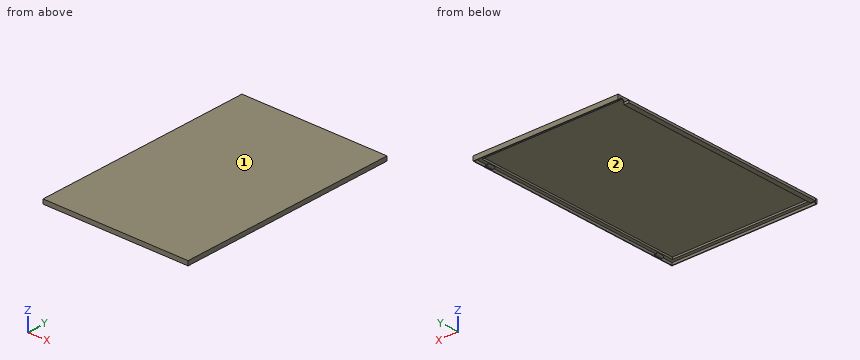
Autodesk Inventor part; units mm, degrees
ref_plane "DPB21_XY" through (247.5, 377.5, 0) normal (0, 0, 1) x (1, 0, 0)
ref_plane "DPB21_YZ" through (247.5, 377.5, 0) normal (1, 0, 0) x (0, 1, 0)
ref_plane "DPB21_ZX" through (247.5, 377.5, 0) normal (0, 1, 0) x (0, 0, 1)
sketch "Skizze_1" plane through (0, 0, 0) normal (0, 0, 1) x (1, 0, 0)
  line L0 (-247.5, 377.5) -> (-247.5, -377.5)
  line L1 (-247.5, -377.5) -> (247.5, -377.5)
  line L2 (247.5, -377.5) -> (247.5, 377.5)
  line L3 (247.5, 377.5) -> (-247.5, 377.5)
extrude "Extrusion1" add sketch "Skizze_1" against normal blind 15
sketch "Skizze_2" plane through (0, 0, 0) normal (1, 0, 0) x (0, 0, -1)
  line L0 (2, 375.5) -> (2, -375.5)
  line L1 (2, -375.5) -> (17, -375.5)
  line L2 (17, -375.5) -> (17, 375.5)
  line L3 (17, 375.5) -> (2, 375.5)
extrude "Extrusion2" cut sketch "Skizze_2" along normal mid plane 491
sketch "Skizze_3" plane through (0, 0, -2) normal (0, 0, 1) x (1, 0, 0)
  line L0 (-245.5, 361.5) -> (231.5, 361.5)
  line L1 (231.5, 361.5) -> (231.5, -361.5)
  line L2 (231.5, -361.5) -> (-245.5, -361.5)
  line L3 (-245.5, -361.5) -> (-245.5, -373.5)
  line L4 (-245.5, -373.5) -> (243.5, -373.5)
  line L5 (243.5, -373.5) -> (243.5, 373.5)
  line L6 (243.5, 373.5) -> (-245.5, 373.5)
  line L7 (-245.5, 373.5) -> (-245.5, 361.5)
sketch "Skizze_21" plane through (0, -320.6, 0) normal (0, 1, 0) x (1, 0, 0)
  arc A0 (240, 12.35) -> (240, 4.05) centre (240, 8.2) ccw
  line L0 (240, 4.05) -> (245.5, 4.05)
  line L1 (245.5, 4.05) -> (245.5, 5.5)
  line L2 (245.5, 5.5) -> (240, 5.5)
  arc A1 (240, 10.9) -> (240, 5.5) centre (240, 8.2) ccw
  line L3 (240, 10.9) -> (245.5, 10.9)
  line L4 (245.5, 10.9) -> (245.5, 12.35)
  line L5 (245.5, 12.35) -> (240, 12.35)
extrude "Extrusion3" add sketch "Skizze_21" along normal mid plane 26
sketch "Skizze_22" plane through (0, 320.6, 0) normal (0, 1, 0) x (1, 0, 0)
  arc A0 (240, 12.35) -> (240, 4.05) centre (240, 8.2) ccw
  line L0 (240, 4.05) -> (245.5, 4.05)
  line L1 (245.5, 4.05) -> (245.5, 5.5)
  line L2 (245.5, 5.5) -> (240, 5.5)
  arc A1 (240, 10.9) -> (240, 5.5) centre (240, 8.2) ccw
  line L3 (240, 10.9) -> (245.5, 10.9)
  line L4 (245.5, 10.9) -> (245.5, 12.35)
  line L5 (245.5, 12.35) -> (240, 12.35)
extrude "Extrusion4" add sketch "Skizze_22" along normal mid plane 26
sketch "Skizze_23" plane through (0, 0, 0) normal (0, 1, 0) x (1, 0, 0)
  line L0 (-263.5, 19) -> (-248, 19)
  arc A0 (-247.5, 18.5) -> (-248, 19) centre (-248, 18.5) ccw
  line L1 (-247.5, 18.5) -> (-247.5, 15)
  line L2 (-247.5, 15) -> (-245.5, 15)
  line L3 (-245.5, 15) -> (-245.5, 19.5)
  arc A1 (-245.5, 19.5) -> (-247, 21) centre (-247, 19.5) ccw
  line L4 (-247, 21) -> (-263.5, 21)
  line L5 (-263.5, 21) -> (-263.5, 19)
extrude "Extrusion5" add sketch "Skizze_23" along normal mid plane 707
sketch "Skizze_24" plane through (-247.5, 0, 0) normal (1, 0, 0) x (0, 0, -1)
  arc A0 (13.25, 372.2142) -> (15.5, 354.5) centre (15.5, 363.5) ccw
  line L0 (15.5, 354.5) -> (15.5, 375.119)
  arc A1 (13.25, 372.2142) -> (15.5, 375.119) centre (12.5, 375.119) ccw
extrude "Extrusion6" cut sketch "Skizze_24" along normal blind 3
sketch "Skizze_26" plane through (-247.5, 0, 0) normal (1, 0, 0) x (0, 0, -1)
  arc A0 (15.5, -354.5) -> (13.25, -372.2142) centre (15.5, -363.5) ccw
  arc A1 (15.5, -375.119) -> (13.25, -372.2142) centre (12.5, -375.119) ccw
  line L0 (15.5, -375.119) -> (15.5, -354.5)
extrude "Extrusion7" cut sketch "Skizze_26" along normal blind 3
sketch "Skizze_27" plane through (0, 0, 0) normal (0, 1, 0) x (1, 0, 0)
  line L0 (-263.5, 19) -> (-263.5, 13)
  line L1 (-263.5, 13) -> (-247.5, 13)
  line L2 (-247.5, 13) -> (-247.5, 19)
  line L3 (-247.5, 19) -> (-263.5, 19)
extrude "Extrusion8" add sketch "Skizze_27" along normal mid plane 707
extrude "Extrusion9" add sketch "Skizze_3" against normal blind 6.5
ref_plane "DPB21_XY" through (247.5, 377.5, 0) normal (0, 0, 1) x (1, 0, 0)
ref_plane "DPB21_YZ" through (247.5, 377.5, 0) normal (1, 0, 0) x (0, 1, 0)
ref_plane "DPB21_ZX" through (247.5, 377.5, 0) normal (0, 1, 0) x (0, 0, 1)
ref_plane "DPB211_XY" through (250, 377.5, 0) normal (0, 0, 1) x (1, 0, 0)
ref_plane "DPB211_YZ" through (250, 377.5, 0) normal (1, 0, 0) x (0, 1, 0)
ref_plane "DPB211_ZX" through (250, 377.5, 0) normal (0, 1, 0) x (0, 0, 1)
ref_plane "DPB22_XY" through (-247.5, 377.5, 0) normal (0, 0, 1) x (1, 0, 0)
ref_plane "DPB22_YZ" through (-247.5, 377.5, 0) normal (1, 0, 0) x (0, 1, 0)
ref_plane "DPB22_ZX" through (-247.5, 377.5, 0) normal (0, 1, 0) x (0, 0, 1)
ref_plane "DPB41_XY" through (205.5, 349, 0) normal (0, 0, 1) x (1, 0, 0)
ref_plane "DPB41_YZ" through (205.5, 349, 0) normal (1, 0, 0) x (0, 1, 0)
ref_plane "DPB41_ZX" through (205.5, 349, 0) normal (0, 1, 0) x (0, 0, 1)
ref_plane "DPB42_XY" through (-218.5, 299, 0) normal (0, 0, 1) x (1, 0, 0)
ref_plane "DPB42_YZ" through (-218.5, 299, 0) normal (1, 0, 0) x (0, 1, 0)
ref_plane "DPB42_ZX" through (-218.5, 299, 0) normal (0, 1, 0) x (0, 0, 1)
ref_plane "DPB51_XY" through (-224.5, 287.5, 0) normal (0, 0, 1) x (1, 0, 0)
ref_plane "DPB51_YZ" through (-224.5, 287.5, 0) normal (1, 0, 0) x (0, 1, 0)
ref_plane "DPB51_ZX" through (-224.5, 287.5, 0) normal (0, 1, 0) x (0, 0, 1)
ref_plane "DPB52_XY" through (211.5, 337.5, 0) normal (0, 0, 1) x (1, 0, 0)
ref_plane "DPB52_YZ" through (211.5, 337.5, 0) normal (1, 0, 0) x (0, 1, 0)
ref_plane "DPB52_ZX" through (211.5, 337.5, 0) normal (0, 1, 0) x (0, 0, 1)
ref_plane "tuer_XY" through (240, -320.6, -8.2) normal (0, 1, 0) x (1, 0, 0)
ref_plane "tuer_YZ" through (240, -320.6, -8.2) normal (1, 0, 0) x (0, 0, -1)
ref_plane "tuer_ZX" through (240, -320.6, -8.2) normal (0, 0, -1) x (0, 1, 0)
ref_plane "tuer_l_XY" through (240, 320.6, -8.2) normal (0, 1, 0) x (1, 0, 0)
ref_plane "tuer_l_YZ" through (240, 320.6, -8.2) normal (1, 0, 0) x (0, 0, -1)
ref_plane "tuer_l_ZX" through (240, 320.6, -8.2) normal (0, 0, -1) x (0, 1, 0)
properties part number "1130_01_02 (2)"
Build history of the part. All positions in model axes, mm. Face numbers are marked on the shaded views. Coordinates: 2 decimals unless noted, no trailing zeros. Order: outer loops, then holes, each group sorted by start corner. A loop starts at its lowest first (then second) coordinate and runs counter-clockwise, first axis right, second up. Notation, with made-up numbers: (29.25, -18.75) -> (85.25, -18.75) arc R9 cw to (85.25, -14.75) -> close; hole circle Ø9 at (5, 67). An arc over 180 degrees is marked (long way). Answer in a Markdown table with one row per item. Add a question column.
Q1. Mould opens along X. For the marked faces 1 and 2 say: +X half, -X half, draft (parallel to the pull), parting line (faces both ways), or undercut.
Q2. Drop flat-ended pins along their axis: pin 1 (4.5 mm diameter, centred on y = -154.5, z = -9, fed in from -X); pin 2 (3 mm diameter, centred on x = 243, y = -318, fed in from -Z); pin 3 (0.8 mm diameter, centred on x = -247, y = -354, fed in from -Z). Give the stop position or say it passes through.
Q3. Band-saw the part on C-C, the plane y = 203.5. List the corners of the cut face in (x, z), then the cut area to 3 significant figures.
Q4. Band-saw the part on A-A, the plane y = -319. List the corners of the cut face in (x, z), then the cut area to 3 significant figures.
Q5. Wall check: line 1 along Y through (x, z) = (173, -5.25); line 2 along X through (y, z) = (62.5, -6.25); line 3 along X through (y, z) = (172, -13.75). Give the ranges that are in metal, low to high. Write a range as [from, to].
Q6. Band-saw the part on B-B, the plane x = -207.5. List the corners of the cut face in (y, z), then the cut area to 3 significant figures.
Answers follow:
| question | item | result |
|---|---|---|
| 1 | face 1 | draft |
| 1 | face 2 | undercut |
| 2 | pin 1 | x = -247.5 |
| 2 | pin 2 | z = -12.35 |
| 2 | pin 3 | z = -15 |
| 3 | outline | (-263.5, -21) -> (-247, -21) arc R1.5 ccw to (-245.5, -19.5) -> (-245.5, -2) -> (231.5, -2) -> (231.5, -8.5) -> (243.5, -8.5) -> (243.5, -2) -> (245.5, -2) -> (245.5, -15) -> (247.5, -15) -> (247.5, 0) -> (-247.5, 0) -> (-247.5, -13) -> (-263.5, -13) -> close |
| 3 | area | 1,260 mm^2 |
| 4 | outline | (-263.5, -21) -> (-247, -21) arc R1.5 ccw to (-245.5, -19.5) -> (-245.5, -2) -> (231.5, -2) -> (231.5, -8.5) -> (235.86, -8.5) arc R4.15 ccw to (240, -12.35) -> (245.5, -12.35) -> (245.5, -15) -> (247.5, -15) -> (247.5, 0) -> (-247.5, 0) -> (-247.5, -13) -> (-263.5, -13) -> close; hole (237.32, -8.5) arc R2.7 ccw to (240, -10.9) -> (245.5, -10.9) -> (245.5, -5.5) -> (243.5, -5.5) -> (243.5, -8.5) -> close; hole (243.5, -4.05) -> (245.5, -4.05) -> (245.5, -2) -> (243.5, -2) -> close |
| 4 | area | 1,280 mm^2 |
| 5 | line 1 | [-377.5, -375.5], [-373.5, -361.5], [361.5, 373.5], [375.5, 377.5] |
| 5 | line 2 | [-247.5, -245.5], [231.5, 243.5], [245.5, 247.5] |
| 5 | line 3 | [-263.5, -245.5], [245.5, 247.5] |
| 6 | outline | (-377.5, -15) -> (-375.5, -15) -> (-375.5, -2) -> (-373.5, -2) -> (-373.5, -8.5) -> (-361.5, -8.5) -> (-361.5, -2) -> (361.5, -2) -> (361.5, -8.5) -> (373.5, -8.5) -> (373.5, -2) -> (375.5, -2) -> (375.5, -15) -> (377.5, -15) -> (377.5, 0) -> (-377.5, 0) -> close |
| 6 | area | 1,720 mm^2 |
